```python
from build123d import *

# Parameters (mm, degrees)
BOSS_EXTRUDE1_DEPTH = 9.9
SKETCH4_W           = 5.781088914
SKETCH4_H           = 1
SKETCH4_W_2         = 5.781088913
CUT_EXTRUDE3_DEPTH  = 20.352504887


with BuildPart() as part:
    # Sketch1 → Boss-Extrude1 (new body)
    with BuildSketch(Plane.XY):
        with BuildLine():
            Line((3.052327113, 5.893513233), (12.052327113, 5.893513233))
            ThreePointArc((12.052327113, 5.893513233), (13.802327113, 5.424602146), (15.083416026, 4.143513233))
            add(Edge.make_bspline(
                [(14.357213227, 3.893513233), (14.754135226, 3.935799795), (15.083416026, 4.143513233)],
                knots=[0, 0, 0, 1, 1, 1], degree=2))
            ThreePointArc((14.357213227, 3.893513233), (9.302327113, 2.393513233), (14.357213227, 0.893513233))
            add(Edge.make_bspline(
                [(14.357213227, 0.893513233), (14.754135226, 0.851226671), (15.083416026, 0.643513233)],
                knots=[0, 0, 0, 1, 1, 1], degree=2))
            ThreePointArc((15.083416026, 0.643513233), (13.802327113, -0.637575681), (12.052327113, -1.106486767))
            Line((12.052327113, -1.106486767), (3.052327113, -1.106486767))
            ThreePointArc((3.052327113, -1.106486767), (1.302327113, -0.637575681), (0.021238199, 0.643513233))
            add(Edge.make_bspline(
                [(0.747440998, 0.893513233), (0.350518999, 0.851226671), (0.021238199, 0.643513233)],
                knots=[0, 0, 0, 1, 1, 1], degree=2))
            ThreePointArc((0.747440998, 0.893513233), (5.802327113, 2.393513233), (0.747440998, 3.893513233))
            add(Edge.make_bspline(
                [(0.747440998, 3.893513233), (0.350518999, 3.935799795), (0.021238199, 4.143513233)],
                knots=[0, 0, 0, 1, 1, 1], degree=2))
            ThreePointArc((0.021238199, 4.143513233), (1.302327113, 5.424602146), (3.052327113, 5.893513233))
        make_face()
    extrude(amount=BOSS_EXTRUDE1_DEPTH)

    # Sketch4 → Cut-Extrude3 (cut, through all)
    with BuildSketch(Plane(origin=(0, 5.893513233, 0), x_dir=(1, 0, 0), z_dir=(0, 1, 0))):
        with Locations((2.911782656, -3.1)):
            Rectangle(SKETCH4_W, SKETCH4_H)
        with Locations((12.192871569, -3.1)):
            Rectangle(SKETCH4_W_2, SKETCH4_H)
        with Locations((12.192871569, -6.8)):
            Rectangle(SKETCH4_W_2, SKETCH4_H)
        with Locations((2.911782656, -6.8)):
            Rectangle(SKETCH4_W, SKETCH4_H)
    extrude(amount=-CUT_EXTRUDE3_DEPTH, mode=Mode.SUBTRACT)


solid = part.part
```
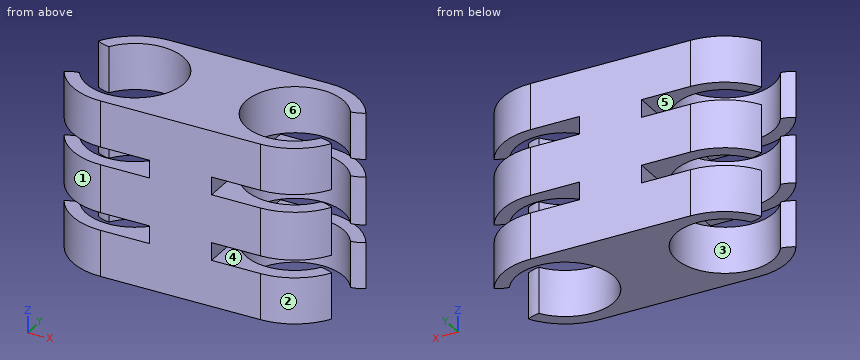
Geometry check sheet. Reference: the model listing, model coordinates, mm. Face numbers are marked on the shaded views. A direction names the side the tool comes from. Give positions to 0.01 mm unless a question says otherwise; leave off trailing zeros. Loops run counter-clockwise (first coordinate to the right, second up) from the corner with the lowest first, then second, coordinate; pieces in that order, holes last. Notation, with made-up numbers: (-2, 59.5) - (43, 59.5) arc R25 ccw to (43, 88.5) - close; hole circle Ø6 at (18.5, -15). An arc over 180 degrees is marked (long way). Use CSV: the item, a comma, the result in double quotes. Start each with the question number.
Q1. Section check C-C, the plane x = 3.25. Record the cut outline in (y, z), and give its area (3 significant figures).
Q2. Section check B-B, the plane y = 1.5. Record the cut outline in (x, z), and give its area (3 significant figures).
Q3. Go/stop test with flat-tipped pins: pin 1 Ø1.1 at (x, y) = (13.5, 0.5) entering from -Z; pin 2 Ø1.1 at (y, z) = (1.5, 3) entering from -X; pin 3 Ø2 at (y, z) = (2.5, 7.5) entering from +X. Record where each tip stops, or that it passes through.
Q4. Release check for a two-part mould opening along X. For the marked faces 1, 2 and 3 record: +X half, -X half, draft (parallel to the pull), parting line (faces both ways), or undercut.
Q5. Access from +Z, -Z, +X, -X, +Y, -Y to the whole of each face (thin tool, end or side, straight path). Record for the marked faces 4, 5 and 6.
Q6. Scan lines: probe 1 along X at (y, z) = (0, 2.25); probe 2 along Y at (x, z) = (3, 1.25); probe 3 along X at (y, z) = (4.75, 1.25). Record each from-to range of solid material in increasing order. Write a range as from..to.
Q7. Section check A-A, the plane x = 11. Record the cut outline in (y, z).
Q8. Section check D-D, the plane z = 6.5. Record the cut outline in (x, y).
Findings below:
1,outline,"(-1.11, 0) - (-0.35, 0) - (-0.35, 2.6) - (-1.11, 2.6) - close; (-1.11, 3.6) - (-0.35, 3.6) - (-0.35, 6.3) - (-1.11, 6.3) - close; (-1.11, 7.3) - (-0.35, 7.3) - (-0.35, 9.9) - (-1.11, 9.9) - close; (5.14, 0) - (5.89, 0) - (5.89, 2.6) - (5.14, 2.6) - close; (5.14, 3.6) - (5.89, 3.6) - (5.89, 6.3) - (5.14, 6.3) - close; (5.14, 7.3) - (5.89, 7.3) - (5.89, 9.9) - (5.14, 9.9) - close"
1,area,"12.0 mm^2"
2,outline,"(5.65, 0) - (9.45, 0) - (9.45, 2.6) - (9.3, 2.6) - (9.3, 3.6) - (9.45, 3.6) - (9.45, 6.3) - (9.3, 6.3) - (9.3, 7.3) - (9.45, 7.3) - (9.45, 9.9) - (5.65, 9.9) - (5.65, 7.3) - (5.8, 7.3) - (5.8, 6.3) - (5.65, 6.3) - (5.65, 3.6) - (5.8, 3.6) - (5.8, 2.6) - (5.65, 2.6) - close"
2,area,"37.0 mm^2"
3,pin 1,"stops at z = 0"
3,pin 2,"stops at x = 5.49"
3,pin 3,"stops at x = 9.53"
4,face 1,"-X half"
4,face 2,"+X half"
4,face 3,"undercut"
5,face 4,"+X, +Y, -Y"
5,face 5,"-X, +Y, -Y"
5,face 6,"+Z, -Z"
6,probe 1,"x = 0.5..1.7, 4.41..10.7, 13.41..14.61"
6,probe 2,"y = -1.11..-0.36, 5.14..5.89"
6,probe 3,"x = 0.46..1.63, 4.47..10.63, 13.47..14.64"
7,outline,"(-1.11, 0) - (-0.15, 0) - (-0.15, 2.6) - (-1.11, 2.6) - close; (-1.11, 3.6) - (-0.15, 3.6) - (-0.15, 6.3) - (-1.11, 6.3) - close; (-1.11, 7.3) - (-0.15, 7.3) - (-0.15, 9.9) - (-1.11, 9.9) - close; (4.93, 0) - (5.89, 0) - (5.89, 2.6) - (4.93, 2.6) - close; (4.93, 3.6) - (5.89, 3.6) - (5.89, 6.3) - (4.93, 6.3) - close; (4.93, 7.3) - (5.89, 7.3) - (5.89, 9.9) - (4.93, 9.9) - close"
8,outline,"(5.8, -1.11) - (9.3, -1.11) - (9.3, 5.89) - (5.8, 5.89) - close"
